The model under review builds one solid part; all positions refer to its coordinate system, in mm. A direction names the side the tool comes from. Coordinates: 2 decimals unless noted, no trailing zeros. Write each loop counter-clockwise with the first axis right and the second up, starting at its lowest first coordinate (ties: lowest second). Pieces come first, ordered by that corner, then holes.
1) Add section D-D, the plane y = 0. State the section outline as (x, z) points (1 decimal).
2) Add section C-C, the plane x = 0. State the section outline as (y, z) points (1 decimal), then the cut area to 3 significant figures.
3) Add section A-A, the plane x = 38.1. State the section outline as (y, z) points (1 decimal), then the cut area to 3 significant figures.
4) Machinability: for faces 5 (the flat face through (32, -12.065, 2)), 6 (the cylindrical face through (-0.42, -66.71, 1.57)), which of the approach directions +Z, -Z, +X, -X, +Y, -Y give a long, thin tool a straight path to every point of the face, cutting with its end or side? Answer none if there is none.
5) Mouldability with a two-part tool opening along Y and no side actions: class faces 1 (the flat face through (12.065, -45, 2)), 2 (the flat face through (0, -76.835, 2)), 3 (the cylindrical face through (-0.7, -34.94, 1.57)), 4 (the cylindrical face through (-10.16, 10.25, 1.61)) as released by +Y, released by -Y, zero draft, split by the parting line, or undercut.
6) For P1, Ø10.5, axis at x = 38.1, y = 0, coming from the +Z side (3 decimals); P2, Ø4, axis at x = 0, y = -63.5, coming from the -Z side (3 decimals); P3, Ø1.6, axis at y = -36, z = 1.5, coming from the +X side (3 decimals), all flat-tipped, find the tip position at first contact; note any pin that passes through.
7) For line 1 (Y direction, x = 0, z = 1.65) (1 decimal); line 2 (Y direction, x = 2.5, z = 0.85) (3 decimals); line 3 (X direction, y = -32.5, z = 1.3) (3 decimals), list the stretches that pass through material, from the lowest coordinate up.
Autodesk Fusion 360 part; units mm, degrees
sketch "Sketch1" plane through (0, 0, 0) normal (0, 0, 1) x (1, 0, 0)
  circle A0 centre (0, -38.1) radius 3.2385
  circle A1 centre (0, -63.5) radius 3.2385
  circle A2 centre (12.7, 0) radius 3.2385
  circle A3 centre (38.1, 0) radius 3.2385
  line L0 (-12.065, 12.065) -> (-12.065, -76.835)
  line L1 (-12.065, -76.835) -> (12.065, -76.835)
  line L2 (12.065, -76.835) -> (12.065, -12.065)
  line L3 (12.065, -12.065) -> (51.435, -12.065)
  line L4 (51.435, -12.065) -> (51.435, 12.065)
  line L5 (51.435, 12.065) -> (-12.065, 12.065)
  line L6 (0, 0) -> (51.435, 0) construction
  line L7 (0, 0) -> (0, -76.835) construction
  dimension "d1" = 6.477
  dimension "d2" = 38.1
  dimension "d4" = 25.4
  dimension "d6" = 12.7
  dimension "d8" = 24.13
  dimension "d9" = 24.13
  dimension "d10" = 88.9
  dimension "d11" = 25.4
  dimension "d12" = 63.5
extrude "Extrude1" add sketch "Sketch1" along normal blind 3.175
fillet "Fillet1" radius 6.35 6 edges at (12.065, -76.835, 1.5875) (-12.065, -76.835, 1.5875) (-12.065, 12.065, 1.5875) (51.435, -12.065, 1.5875) (51.435, 12.065, 1.5875) (12.065, -12.065, 1.5875)
equation "d13 = ( 1 / 8 ) * 1 in"
Geometry results:
1. outline: (-12.1, 0) - (9.5, 0) - (9.5, 3.2) - (-12.1, 3.2) - close; (15.9, 0) - (34.9, 0) - (34.9, 3.2) - (15.9, 3.2) - close; (41.3, 0) - (51.4, 0) - (51.4, 3.2) - (41.3, 3.2) - close
2. outline: (-76.8, 0) - (-66.7, 0) - (-66.7, 3.2) - (-76.8, 3.2) - close; (-60.3, 0) - (-41.3, 0) - (-41.3, 3.2) - (-60.3, 3.2) - close; (-34.9, 0) - (12.1, 0) - (12.1, 3.2) - (-34.9, 3.2) - close
2. area: 241 mm2
3. outline: (-12.1, 0) - (-3.2, 0) - (-3.2, 3.2) - (-12.1, 3.2) - close; (3.2, 0) - (12.1, 0) - (12.1, 3.2) - (3.2, 3.2) - close
3. area: 56.0 mm2
4. face 5: +Z, -Z, +X, -Y
4. face 6: +Z, -Z
5. face 1: zero draft
5. face 2: released by -Y
5. face 3: undercut
5. face 4: released by +Y
6. P1: stops at z = 3.175
6. P2: passes through
6. P3: stops at x = 12.065
7. line 1: y = -76.8 to -66.7, -60.3 to -41.3, -34.9 to 12.1
7. line 2: y = -76.835 to -65.559, -61.441 to -40.159, -36.041 to 12.065
7. line 3: x = -12.065 to 12.065
